Part model, mm, in its own coordinate system. Coordinates: 2 decimals unless noted, no trailing zeros. Answer as a JSON object with one key per item and string values. Group by question number.
1. Drop a flat-ended pin along its axis: pin 1 Ø2.5 at (x, y) = (-7.49, -212.22) entering from -Z. Give the stop position or say it passes through.
2. Mould opens along Y. For faces 1 (the face through (-8, -101, 1.905)), 2 (the face through (-7.397, -214.442, 0.939)) say: released by +Y, released by -Y, zero draft, split by the parting line, or undercut.
3. Drill centre lines: L1, parallel to Y at x = -7.5, z = 0.55; L2, parallel to Y at x = -6.5, z = 0.6. Where is each one in solid material? Low to high.
Autodesk Inventor part; units mm, degrees
ref_plane "Work Plane1" through (-19.7981, -102.6844, 0) normal (0, 1, 0) x (1, 0, 0)
ref_plane "YZ Plane" through (0, 0, 0) normal (1, 0, 0) x (0, 1, 0)
ref_plane "XZ Plane" through (0, 0, 0) normal (0, 1, 0) x (-1, 0, 0)
sketch "Sketch1" plane through (0, 0, 0) normal (0, 0, 1) x (1, 0, 0)
  line L0 (-19.7981, 13.2031) -> (4.8082, 13.2031)
  line L1 (4.8082, 13.2031) -> (4.8082, -218.5719)
  line L2 (4.8082, -218.5719) -> (-19.7981, -218.5719)
  line L3 (-19.7981, -218.5719) -> (-19.7981, 13.2031)
  point P0 (0, 0)
  dimension "d0" = 231.775
  dimension "d1" = 24.6062
extrude "Extrusion1" add sketch "Sketch1" along normal blind 1.905
sketch "Sketch2" plane through (0, 0, 1.905) normal (0, 0, 1) x (1, 0, 0)
  line L0 (4.8082, 13.2031) -> (-19.7981, 13.2031)
  line L1 (-7.4949, 13.2031) -> (-7.4949, -18.5655)
  line L2 (-19.7981, 13.2031) -> (-19.7981, -218.5719)
  line L3 (4.8082, -218.5719) -> (4.8082, 13.2031)
  line L4 (-19.7981, 6.8531) -> (4.8082, 6.8531)
  point P0 (0, 0)
  point P1 (-7.4949, 6.8531)
  point P2 (-7.4949, 6.8531)
  point P3 (-7.4949, 6.8531)
  dimension "d4" = 12.3031
  dimension "d6" = 6.35
hole "Hole1" at (-7.4949, 6.8531, 1.905) direction (0, 0, -1) diameter 4.445 end through all
sketch "Sketch3" plane through (0, 0, 1.905) normal (0, 0, 1) x (1, 0, 0)
  line L0 (4.8082, 13.2031) -> (4.8082, -218.5719)
  line L1 (4.8082, -102.6844) -> (-19.7981, -102.6844)
  line L2 (-19.7981, -218.5719) -> (-19.7981, 13.2031)
  line L3 (4.8082, 13.2031) -> (-19.7981, 13.2031)
  line L4 (4.8082, -218.5719) -> (4.8082, 13.2031)
  point P0 (0, 0)
  dimension "d14" = 231.775
  dimension "d15" = 115.8875
ref_plane "Work Plane1" through (-19.7981, -102.6844, 0) normal (0, 1, 0) x (1, 0, 0)
mirror "Mirror1" about plane through (-19.7981, -102.6844, 0) normal (0, 1, 0) of "Hole1"
equation "\"d15\" = 0.5 * d14"
properties part number "Rotation Resistor-01"
Outcome:
{
 "1": {"pin 1": "passes through"},
 "2": {"face 1": "zero draft", "face 2": "undercut"},
 "3": {"L1": "y = -218.57 to -214.44, -210 to 4.63, 9.08 to 13.2", "L2": "y = -218.57 to -214.21, -210.23 to 4.87, 8.84 to 13.2"}
}
